CAD build for the part. Positions are in the model's coordinates, mm. A direction names the side the tool comes from. Give positions to 0.01 mm unless a question says otherwise; leave off trailing zeros. Loops run counter-clockwise (first coordinate to the right, second up) from the corner with the lowest first, then second, coordinate; pieces in that order, holes last.
Item 1: Saw through at A-A on z = 0. Give the cut face in (x, y), plus the area to 3 significant figures.
Item 2: Mould opens along X. For faces 1 (the cylindrical face through (46.37, 14.3, 10.3)), 2 (the cylindrical face through (-8.66, 15.93, -0.03)), 3 (the flat face through (-1, 29, -10)) say: released by +X, released by -X, zero draft, split by the parting line, or undercut.
Item 3: Which spindle directions (+Z, -Z, +X, -X, +Y, -Y) get a long thin tool onto all of the face, cutting with end or side? Do faces 4 (the flat face through (4, 2.482, 7)), 5 (the flat face through (-1, 0, -10)). Say none if no direction does.
Item 4: Drop flat-ended pins along their axis: P1, Ø3, axis at x = 36.5, y = 12.5, coming from the +Z side; P2, Ø2, axis at x = 8.5, y = 19.5, coming from the +Z side; P3, Ø0.7, axis at x = -8, z = 0, coming from the +Y side. Give the stop position or say it passes through.
Item 5: Saw through at B-B on x = 0. Give the cut face in (y, z).
Item 6: Saw through at C-C on y = 11.75. Give the cut face in (x, z).
Item 7: Saw through at D-D on z = -41. Give the cut face in (x, y), plus the area to 3 significant figures.
Item 8: Probe probe 1 along X at (y, z) = (17, 0); probe 2 along X at (y, z) = (17.75, -4); probe 3 along X at (y, z) = (7, -37). List the from-to ranges inside material, lowest first.
from build123d import *

# Parameters (mm, degrees)
SKETCH1_R           = 47.5
BOSS_EXTRUDE1_DEPTH = 29
SKETCH2_R           = 7.5
CUT_EXTRUDE1_DEPTH  = 74.167615787
SKETCH3_R           = 1.533548882
CUT_EXTRUDE2_DEPTH  = 26.517871
CIRPATTERN1_START   = 2.482128874
CIRPATTERN1_DEPTH   = 26.517871126


# Read off the part's stored shape, not the designer's step: CirPattern1
with BuildPart() as part:
    # Sketch1 → Boss-Extrude1 (new body)
    with BuildSketch(Plane(origin=(0, 0, 0), x_dir=(1, 0, 0), z_dir=(0, 1, 0))):
        with Locations(Location((0, 0, 0), (0, 0, 90))):
            Circle(SKETCH1_R)
    extrude(amount=BOSS_EXTRUDE1_DEPTH)

    # Sketch2 → Cut-Extrude1 (cut, through all)
    with BuildSketch(Plane(origin=(0, 0, 0), x_dir=(1, 0, 0), z_dir=(0, 1, 0))):
        with Locations(Location((0, 0, 0), (0, 0, 90))):
            Circle(SKETCH2_R)
    extrude(amount=CUT_EXTRUDE1_DEPTH, mode=Mode.SUBTRACT)

    # Sketch3 → Cut-Extrude2 (cut)
    with BuildSketch(Plane(origin=(0, 29, 0), x_dir=(1, 0, 0), z_dir=(0, 1, 0))):
        with Locations((-7.124914208, 0)):
            Circle(SKETCH3_R)
    extrude(amount=-CUT_EXTRUDE2_DEPTH, mode=Mode.SUBTRACT)

    # CirPattern1 outline → CirPattern1 (cut)
    with BuildSketch(Plane(origin=(0, 0, 0), x_dir=(1, 0, 0), z_dir=(0, 1, 0)).offset(CIRPATTERN1_START)):
        with BuildLine():
            ThreePointArc((-2.358052174, -7.119662207), (-3.75, -6.495190528), (-4.986782251, -5.60196419))
            ThreePointArc((-4.986782251, -5.60196419), (-4.329231545, -7.498448994), (-2.358052174, -7.119662207))
        make_face()
        with BuildLine():
            ThreePointArc((-2.358052174, 7.119662207), (-4.329231545, 7.498448994), (-4.986782251, 5.60196419))
            ThreePointArc((-4.986782251, 5.60196419), (-3.75, 6.495190528), (-2.358052174, 7.119662207))
        make_face()
        with BuildLine():
            ThreePointArc((4.986782251, -5.60196419), (3.75, -6.495190528), (2.358052174, -7.119662207))
            ThreePointArc((2.358052174, -7.119662207), (4.329231545, -7.498448994), (4.986782251, -5.60196419))
        make_face()
        with BuildLine():
            ThreePointArc((4.986782251, 5.60196419), (4.329231545, 7.498448994), (2.358052174, 7.119662207))
            ThreePointArc((2.358052174, 7.119662207), (3.75, 6.495190528), (4.986782251, 5.60196419))
        make_face()
        with BuildLine():
            ThreePointArc((7.344834425, 1.517698018), (7.5, 0), (7.344834425, -1.517698018))
            ThreePointArc((7.344834425, -1.517698018), (8.65846309, 0), (7.344834425, 1.517698018))
        make_face()
    extrude(amount=CIRPATTERN1_DEPTH, mode=Mode.SUBTRACT)


solid = part.part
Results below:
1. outline: (-47.5, 0) - (-7.5, 0) - (-7.5, 2.48) - (-8.66, 2.48) - (-8.66, 29) - (-47.5, 29) - close; (7.5, 0) - (47.5, 0) - (47.5, 29) - (8.66, 29) - (8.66, 2.48) - (7.5, 2.48) - close
1. area: 2,260 mm2
2. face 1: split by the parting line
2. face 2: undercut
2. face 3: zero draft
3. face 4: +Y
3. face 5: +Z, -Z, +X, -X, -Y
4. P1: stops at z = 32.11
4. P2: stops at z = 46.9
4. P3: stops at y = 2.48
5. outline: (0, -47.5) - (29, -47.5) - (29, -7.5) - (0, -7.5) - close; (0, 7.5) - (29, 7.5) - (29, 47.5) - (0, 47.5) - close
6. outline: circle Ø95 at (0, 0); hole (-7.34, -1.52) arc R7.5 ccw to (-4.99, -5.6) arc R1.53 ccw to (-2.36, -7.12) arc R7.5 ccw to (2.36, -7.12) arc R1.53 ccw to (4.99, -5.6) arc R7.5 ccw to (7.34, -1.52) arc R1.53 ccw to (7.34, 1.52) arc R7.5 ccw to (4.99, 5.6) arc R1.53 ccw to (2.36, 7.12) arc R7.5 ccw to (-2.36, 7.12) arc R1.53 ccw to (-4.99, 5.6) arc R7.5 ccw to (-7.34, 1.52) arc R1.53 ccw to start
7. outline: (-23.98, 0) - (23.98, 0) - (23.98, 29) - (-23.98, 29) - close
7. area: 1,390 mm2
8. probe 1: x = -47.5 to -8.66, 8.66 to 47.5
8. probe 2: x = -47.33 to -6.34, 6.34 to 47.33
8. probe 3: x = -29.79 to 29.79
